from build123d import *

# Parameters (mm, degrees)
F3_DEPTH = 1.6
F4_DEPTH = 1.3
F2_W     = 48.4
F2_H     = 48.4
F5_DEPTH = 1.2


with BuildPart() as f3:
    # F0 (on Top) → F3 (new body)
    with BuildSketch(Plane.XY):
        Polygon((-21.3, 2.314286), (-22.5, 2.314286), (-22.5, -22.885714), (22.5, -22.885714), (22.5, 2.314286), (21.3, 2.314286), (21.3, -21.685714), (-21.3, -21.685714), align=None)
    extrude(amount=F3_DEPTH)

    # F1 (on Top) → F4 (join)
    with BuildSketch(Plane.XY):
        Polygon((22.5, 22.114286), (-22.5, 22.114286), (-22.5, 2.314286), (-21.3, 2.314286), (-21.3, 20.914286), (21.3, 20.914286), (21.3, 2.314286), (22.5, 2.314286), align=None)
    extrude(amount=F4_DEPTH)

    # F2 (on Top) → F5 (join)
    with BuildSketch(Plane.XY):
        with Locations((0, -0.385714)):
            Rectangle(F2_W, F2_H)
        Polygon((-22.5, 2.314286), (-22.5, 22.114286), (22.5, 22.114286), (22.5, 2.314286), (22.5, -22.885714), (-22.5, -22.885714), align=None, mode=Mode.SUBTRACT)
        Polygon((-21.3, 20.914286), (-21.3, 2.314286), (-21.3, -21.685714), (21.3, -21.685714), (21.3, 2.314286), (21.3, 20.914286), align=None)
    extrude(amount=F5_DEPTH)


solid = f3.part
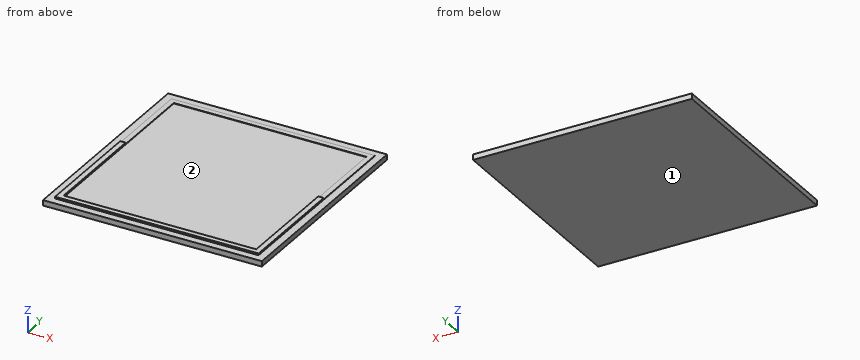
Input: part model. Units: mm. Frame: model coordinates. Face numbers are marked on the shaded views. Coordinates: 2 decimals unless noted, no trailing zeros. Order: outer loops, then holes, each group sorted by start corner. A loop starts at its lowest first (then second) coordinate and runs counter-clockwise, first axis right, second up. Notation, with made-up numbers: M 10,3.25 L 52,3.25 A18 ccw 52,14.25 Z; hole C 13,-37.5 d2. An arc over 180 degrees is marked long. Write item = value, one per line. Start each with the question number.
(1) Pull-direction query (X, two-part tool) for the marked faces 1 and 2; classes: released by +X, released by -X, zero draft, split by the parting line, or undercut.
(2) Section B-B on y = -2. Output: boundary loops of the cut face in (x, z), and give its area (3 significant figures).
(3) First-contact query: P1, Ø4, axis at x = 1, y = -3, coming from the +Z side; P2, Ø2, axis at x = -6.5, y = -5, coming from the -Z side. Flat tips, straight axial feed; report the tip coordinate or a pass-through.
(4) Section A-A on x = 20. Output: boundary loops of the cut face in (y, z), and give its area (3 significant figures).
(5) Line query: line 1 along Y through (x, z) = (4.5, 1.25); line 2 along Z through (x, y) = (5, 8.5); line 3 along Y through (x, z) = (4, 1.4). Output: solid intervals per line, ascending. Write a range as [from, to].
Result set:
q1.face_1 = zero draft
q1.face_2 = undercut
q2.outline = M -24.2,0 L 24.2,0 L 24.2,1.2 L 22.5,1.2 L 22.5,1.6 L 21.3,1.6 L 21.3,1.2 L -21.3,1.2 L -21.3,1.6 L -22.5,1.6 L -22.5,1.2 L -24.2,1.2 Z
q2.area = 59.0 mm²
q3.P1 = 1.2
q3.P2 = 0
q4.outline = M -24.59,0 L 23.81,0 L 23.81,1.2 L 22.11,1.2 L 22.11,1.3 L 20.91,1.3 L 20.91,1.2 L -21.69,1.2 L -21.69,1.6 L -22.89,1.6 L -22.89,1.2 L -24.59,1.2 Z
q4.area = 58.7 mm²
q5.line_1 = [-22.89, -21.69], [20.91, 22.11]
q5.line_2 = [0, 1.2]
q5.line_3 = [-22.89, -21.69]
